Geometry check sheet. Reference: the model listing, model coordinates, mm. A direction names the side the tool comes from. Coordinates: 2 decimals unless noted, no trailing zeros. Loops run counter-clockwise (first coordinate to the right, second up) from the corner with the lowest first, then second, coordinate; pieces in that order, holes last.
from build123d import *

# Parameters (mm, degrees)
SKETCH1_W           = 63.5
SKETCH1_H           = 63.5
SKETCH1_R           = 4.953
BOSS_EXTRUDE1_DEPTH = 3.175


with BuildPart() as part:
    # Sketch1 → Boss-Extrude1 (new body)
    with BuildSketch(Plane.XY):
        Rectangle(SKETCH1_W, SKETCH1_H)
        with Locations((-15.875, 22.06498)):
            Circle(SKETCH1_R, mode=Mode.SUBTRACT)
        with Locations((15.875, 22.06498)):
            Circle(SKETCH1_R, mode=Mode.SUBTRACT)
        with Locations((0, -22.06498)):
            Circle(SKETCH1_R, mode=Mode.SUBTRACT)
        with BuildLine():
            Line((13.97, -25.4), (24.13, -25.4))
            ThreePointArc((24.13, -25.4), (26.035, -27.305), (24.13, -29.21))
            Line((24.13, -29.21), (13.97, -29.21))
            ThreePointArc((13.97, -29.21), (12.065, -27.305), (13.97, -25.4))
        make_face(mode=Mode.SUBTRACT)
        with BuildLine():
            Line((-13.97, -25.4), (-24.13, -25.4))
            ThreePointArc((-24.13, -25.4), (-26.035, -27.305), (-24.13, -29.21))
            Line((-24.13, -29.21), (-13.97, -29.21))
            ThreePointArc((-13.97, -29.21), (-12.065, -27.305), (-13.97, -25.4))
        make_face(mode=Mode.SUBTRACT)
    extrude(amount=BOSS_EXTRUDE1_DEPTH)


solid = part.part
1) Access from +Z, -Z, +X, -X, +Y, -Y to the whole of each face (thin tool, end or side, straight path). Record for faces 1 (the cylindrical face through (-12.065, -27.347, 1.565)), 2 (the flat face through (0, 0, 3.175)).
Data:
face 1: +Z, -Z
face 2: +Z, +X, -X, +Y, -Y
2) Section check D-D on z = 1.9. Record the cut outline in (x, y) (3 decimals), and give its area (3 significant figures).
Data:
outline: (-31.75, -31.75) - (31.75, -31.75) - (31.75, 31.75) - (-31.75, 31.75) - close; hole (-24.13, -29.21) - (-13.97, -29.21) arc R1.905 ccw to (-13.97, -25.4) - (-24.13, -25.4) arc R1.905 ccw to start; hole circle Ø9.906 at (-15.875, 22.065); hole circle Ø9.906 at (0, -22.065); hole circle Ø9.906 at (15.875, 22.065); hole (13.97, -29.21) - (24.13, -29.21) arc R1.905 ccw to (24.13, -25.4) - (13.97, -25.4) arc R1.905 ccw to start
area: 3,700 mm2
3) Material ranges on probe 1 along Y at (x, z) = (-22.5, 0.75); probe 2 along Y at (x, z) = (0, 2.35); probe 3 along X at (y, z) = (18.5, 0.4), recorded low to high.
Data:
probe 1: y = -31.75 to -29.21, -25.4 to 31.75
probe 2: y = -31.75 to -27.02, -17.11 to 31.75
probe 3: x = -31.75 to -19.31, -12.44 to 12.44, 19.31 to 31.75
4) Depth check by flat-ended pin: pin 1 (9 mm diameter, centred on x = 0, y = -22.06, fed in from -Z). Enter the tip coordinate at first touch or a pass-through.
Data:
pin 1: passes through
5) Section check B-B on x = 22.5. Record the cut outline in (y, z) (3 decimals), and give its area (3 significant figures).
Data:
outline: (-31.75, 0) - (-29.21, 0) - (-29.21, 3.175) - (-31.75, 3.175) - close; (-25.4, 0) - (31.75, 0) - (31.75, 3.175) - (-25.4, 3.175) - close
area: 190 mm2
6) Section check A-A on x = 0. Record the cut outline in (y, z) (3 decimals), and give its area (3 significant figures).
Data:
outline: (-31.75, 0) - (-27.018, 0) - (-27.018, 3.175) - (-31.75, 3.175) - close; (-17.112, 0) - (31.75, 0) - (31.75, 3.175) - (-17.112, 3.175) - close
area: 170 mm2
7) Mould release check, pull along Y, two halves, no side actions. Record for faces 3 (the flat face through (-31.75, 0, 2)), 4 (the cylindrical face through (-1.07, -26.9, 1.57)), 5 (the cylindrical face through (-11.3, 20.17, 1.57)), 6 (the flat face through (0, 31.75, 2)): +Y half, -Y half, draft (parallel to the pull), parting line (faces both ways), or undercut.
Data:
face 3: draft
face 4: undercut
face 5: undercut
face 6: +Y half
8) Section check C-C on y = 18. Record the cut outline in (x, z) (3 decimals), and give its area (3 significant figures).
Data:
outline: (-31.75, 0) - (-18.705, 0) - (-18.705, 3.175) - (-31.75, 3.175) - close; (-13.045, 0) - (13.045, 0) - (13.045, 3.175) - (-13.045, 3.175) - close; (18.705, 0) - (31.75, 0) - (31.75, 3.175) - (18.705, 3.175) - close
area: 166 mm2
